Design review of the part shown in the three views and the two pictorial views. Dimensions are in mm from the part's minimum x, y and z. Coordinates: 2 decimals unless noted, no trailing zeros. Write each loop counter-clockwise with the first axis right and the second up, starting at its lowest first coordinate (ties: lowest second). Pieces come first, ordered by that corner, then holes. Notation, with made-up numbers: (-17, 40.25) - (42, 40.25) arc R7 ccw to (42, 46.25) - close; hole circle Ø9 at (-4.75, 18.25). An arc over 180 degrees is marked (long way). Answer as CSV lines item,"result". Start each with the question number.
Q1. For line 1 along Y through (x, z) = (2.1, 0.25); line 2 along Y through (x, z) = (2.4, 0.25) (1 decimal); line 3 along X through (y, z) = (1.5, 0.15), list the stretches that pass through material, from the lowest coordinate up. Write a range as [from, to].
Q2. We need section C-C (x = 4.5). Write out the cut boundary in (y, z).
Q3. We need section A-A (z = 0.4). State how many separate pieces and enclosed holes the cut face has.
Q4. We need section B-B (y = 9). Write out the cut boundary in (x, z).
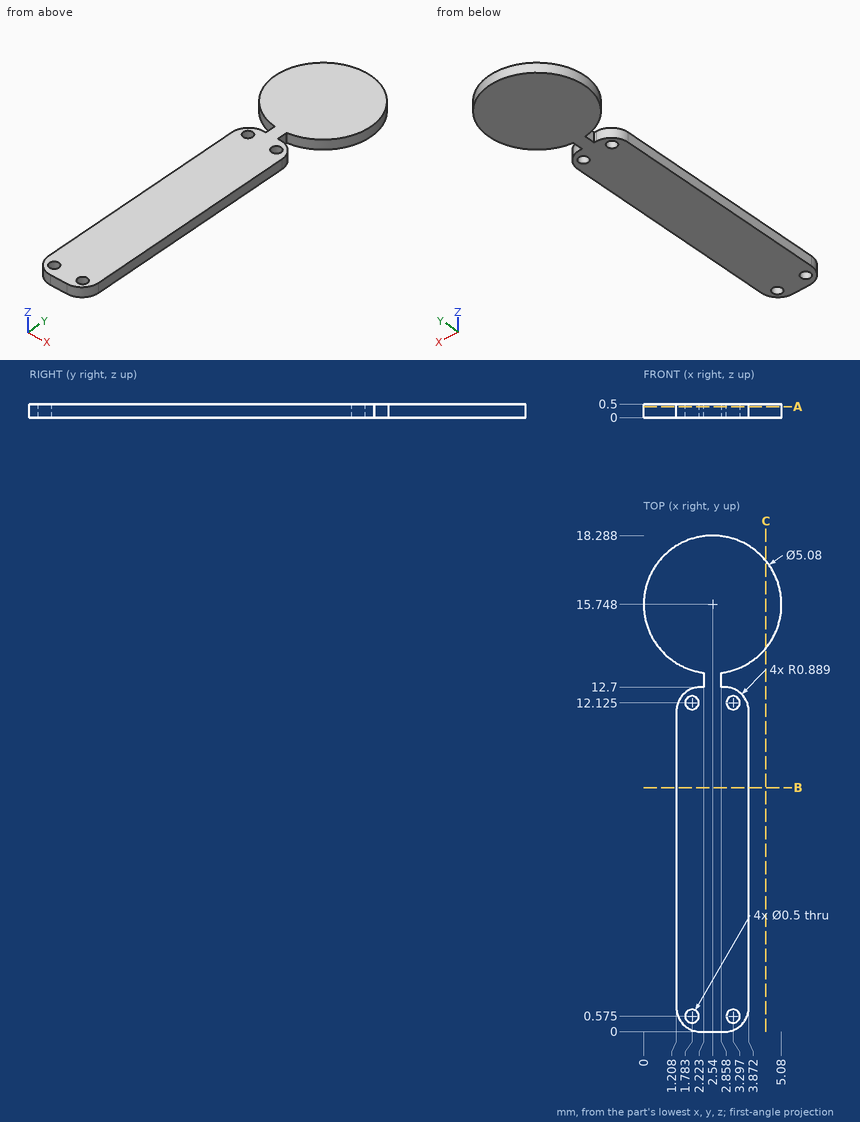
Results list:
1,line 1,"y = [0, 12.7], [13.25, 18.25]"
1,line 2,"y = [0, 18.3]"
1,line 3,"x = [1.21, 3.87]"
2,outline,"(14.13, 0) - (17.36, 0) - (17.36, 0.5) - (14.13, 0.5) - close"
3,separate pieces,"1"
3,enclosed holes,"4"
4,outline,"(1.21, 0) - (3.87, 0) - (3.87, 0.5) - (1.21, 0.5) - close"
